Check sheet for the modelled part. Datum: model origin and axes. Units: mm. A direction names the side the tool comes from. Give positions to 0.01 mm unless a question says otherwise; leave off trailing zeros. Write each loop counter-clockwise with the first axis right and the second up, starting at its lowest first coordinate (ties: lowest second). Pieces come first, ordered by that corner, then holes. Notation, with made-up numbers: M 67,19 L 109,19 A34 ccw 109,56 Z; hole C 66,62.25 d2. An arc over 180 degrees is marked long. Write each question's results on one line, items separated by ' | '. Start each with the question number.
Autodesk Inventor part; units mm, degrees
ref_plane "YZ Plane" through (0, 0, 0) normal (1, 0, 0) x (0, 1, 0)
ref_plane "XZ Plane" through (0, 0, 0) normal (0, 1, 0) x (-1, 0, 0)
ref_plane "XY Plane" through (0, 0, 0) normal (0, 0, 1) x (1, 0, 0)
sketch "Sketch1" plane through (0, 0, 0) normal (0, 1, 0) x (-1, 0, 0)
  line L0 (0.6121, 9.4217) -> (-0.6121, 9.4217)
  line L1 (-3.6121, 6.4217) -> (-3.6121, -6.4217)
  line L2 (-0.6121, -9.4217) -> (0.6121, -9.4217)
  line L3 (3.6121, -6.4217) -> (3.6121, 6.4217)
  line L4 (3.6121, 9.4217) -> (-3.6121, -9.4217) construction
  line L5 (-3.6121, 9.4217) -> (3.6121, -9.4217) construction
  arc A0 (3.6121, 6.4217) -> (0.6121, 9.4217) centre (0.6121, 6.4217) ccw
  arc A1 (-0.6121, 9.4217) -> (-3.6121, 6.4217) centre (-0.6121, 6.4217) ccw
  arc A2 (0.6121, -9.4217) -> (3.6121, -6.4217) centre (0.6121, -6.4217) ccw
  arc A3 (-3.6121, -6.4217) -> (-0.6121, -9.4217) centre (-0.6121, -6.4217) ccw
  line L6 (2.5462, 7.5291) -> (2.5462, -7.1828) construction
  line L7 (2.5462, -7.1828) -> (-2.4754, -7.1828) construction
  line L8 (-2.4754, -7.1828) -> (-2.4754, 7.5291) construction
  line L9 (-2.4754, 7.5291) -> (2.5462, 7.5291) construction
  line L10 (0.1215, 6.8275) -> (0.1215, 5.888)
  spline S0 degree 2 poles (0.1215, 5.888) (0.1215, 5.7568) (0.2446, 5.5598) (0.4744, 5.4573) (0.6385, 5.4573) knots 0 0 0 1 2 3 3 3
  line L11 (0.6385, 5.4573) -> (1.3974, 5.4573)
  spline S1 degree 2 poles (1.3974, 5.4573) (1.5656, 5.4573) (1.8036, 5.5598) (1.9308, 5.7568) (1.9308, 5.888) knots 0 0 0 1 2 3 3 3
  line L12 (1.9308, 5.888) -> (1.9308, 6.8275)
  line L13 (1.9308, 6.8275) -> (2.5462, 6.8275)
  line L14 (2.5462, 6.8275) -> (2.5462, 5.9004)
  spline S2 degree 2 poles (2.5462, 5.9004) (2.5462, 5.5516) (2.2795, 5.0552) (1.7667, 4.7968) (1.4097, 4.7968) knots 0 0 0 1 2 3 3 3
  line L15 (1.4097, 4.7968) -> (0.6179, 4.7968)
  spline S3 degree 2 poles (0.6179, 4.7968) (0.2692, 4.7968) (-0.2313, 5.0593) (-0.4939, 5.5557) (-0.4939, 5.9004) knots 0 0 0 1 2 3 3 3
  line L16 (-0.4939, 5.9004) -> (-0.4939, 6.8275)
  line L17 (-0.4939, 6.8275) -> (0.1215, 6.8275)
  line L18 (2.5462, 7.1886) -> (2.5462, 6.5363)
  line L19 (2.5462, 6.5363) -> (-2.4221, 6.5363)
  line L20 (-2.4221, 6.5363) -> (-2.4221, 7.1886)
  line L21 (-2.4221, 7.1886) -> (2.5462, 7.1886)
  line L22 (2.5462, 3.2173) -> (2.5462, 2.6224)
  line L23 (2.5462, 2.6224) -> (-2.4221, 1.4737)
  line L24 (-2.4221, 1.4737) -> (-2.4221, 2.1711)
  line L25 (-2.4221, 2.1711) -> (1.5287, 2.9219)
  line L26 (1.5287, 2.9219) -> (-2.4221, 3.6685)
  line L27 (-2.4221, 3.6685) -> (-2.4221, 4.366)
  line L28 (-2.4221, 4.366) -> (2.5462, 3.2173)
  line L29 (-0.7277, 3.6316) -> (-0.7277, 2.1588)
  line L30 (-0.7277, 2.1588) -> (-1.339, 2.1588)
  line L31 (-1.339, 2.1588) -> (-1.339, 3.6316)
  line L32 (-1.339, 3.6316) -> (-0.7277, 3.6316)
  spline S4 degree 2 poles (-2.4713, -0.0648) (-2.4713, 0.2962) (-2.2046, 0.8049) (-1.6795, 1.0634) (-1.3062, 1.0634) knots 0 0 0 1 2 3 3 3
  line L33 (-1.3062, 1.0634) -> (2.5462, 1.0634)
  line L34 (2.5462, 1.0634) -> (2.5462, 0.4152)
  line L35 (2.5462, 0.4152) -> (-1.3308, 0.4152)
  spline S5 degree 2 poles (-1.3308, 0.4152) (-1.5769, 0.4152) (-1.8395, 0.169) (-1.8395, -0.0648) knots 0 0 0 1 2 2 2
  spline S6 degree 2 poles (-1.8395, -0.0648) (-1.8395, -0.2987) (-1.5769, -0.5489) (-1.3308, -0.5489) knots 0 0 0 1 2 2 2
  line L36 (-1.3308, -0.5489) -> (2.5462, -0.5489)
  line L37 (2.5462, -0.5489) -> (2.5462, -1.1971)
  line L38 (2.5462, -1.1971) -> (-1.3062, -1.1971)
  spline S7 degree 2 poles (-1.3062, -1.1971) (-1.6795, -1.1971) (-2.2046, -0.9346) (-2.4713, -0.4299) (-2.4713, -0.0648) knots 0 0 0 1 2 3 3 3
  line L39 (2.5462, -1.8494) -> (2.5462, -2.5018)
  line L40 (2.5462, -2.5018) -> (-2.4221, -2.5018)
  line L41 (-2.4221, -2.5018) -> (-2.4221, -1.8494)
  line L42 (-2.4221, -1.8494) -> (2.5462, -1.8494)
  line L43 (-1.8067, -2.1982) -> (-1.8067, -3.913)
  line L44 (-1.8067, -3.913) -> (-2.4221, -3.913)
  line L45 (-2.4221, -3.913) -> (-2.4221, -2.1982)
  line L46 (-2.4221, -2.1982) -> (-1.8067, -2.1982)
  line L47 (2.5462, -5.3366) -> (2.5462, -5.9315)
  line L48 (2.5462, -5.9315) -> (-2.4221, -7.0802)
  line L49 (-2.4221, -7.0802) -> (-2.4221, -6.3828)
  line L50 (-2.4221, -6.3828) -> (1.5287, -5.632)
  line L51 (1.5287, -5.632) -> (-2.4221, -4.8854)
  line L52 (-2.4221, -4.8854) -> (-2.4221, -4.1879)
  line L53 (-2.4221, -4.1879) -> (2.5462, -5.3366)
  line L54 (-0.7277, -4.9223) -> (-0.7277, -6.3951)
  line L55 (-0.7277, -6.3951) -> (-1.339, -6.3951)
  line L56 (-1.339, -6.3951) -> (-1.339, -4.9223)
  line L57 (-1.339, -4.9223) -> (-0.7277, -4.9223)
  point P0 (0, 0)
  dimension "d0" = 3
extrude "Extrusion1" add sketch "Sketch1" against normal blind 2 contours A0 L3 A2 L2 A3 L1 A1 L0 | L17 L16 L19 L20 L21 L18 L13 L12 L10 | L10 L19 L16 L17 | L19 L12 S1 L11 S0 L10 | L10 S0 L11 S1 L12 L19 L14 S2 L15 S3 L16 | L12 L13 L14 L19 | L22 L23 L24 L25 L31 L30 L29 L26 L32 L27 L28 | L31 L32 L29 L26 | L26 L29 L25 L31 | L25 L29 L30 L31 | L26 L25 L29 | S4 L33 L34 L35 S5 S6 L36 L37 L38 S7 | L39 L40 L43 L46 L41 L42 | L43 L44 L45 L40 | L40 L41 L46 L43 | L47 L48 L49 L50 L56 L55 L54 L51 L57 L52 L53 | L56 L57 L54 L51 | L51 L54 L50 L56 | L50 L54 L55 L56 | L51 L50 L54
extrude "Extrusion2" add sketch "Sketch1" along normal blind 1 contours L17 L16 L19 L20 L21 L18 L13 L12 L10 | L10 L19 L16 L17 | L10 S0 L11 S1 L12 L19 L14 S2 L15 S3 L16 | L12 L13 L14 L19 | L22 L23 L24 L25 L31 L30 L29 L26 L32 L27 L28 | L31 L32 L29 L26 | L26 L29 L25 L31 | L25 L29 L30 L31 | S4 L33 L34 L35 S5 S6 L36 L37 L38 S7 | L39 L40 L43 L46 L41 L42 | L43 L44 L45 L40 | L40 L41 L46 L43 | L47 L48 L49 L50 L56 L55 L54 L51 L57 L52 L53 | L56 L57 L54 L51 | L51 L54 L50 L56 | L50 L54 L55 L56
sketch "Sketch2" plane through (0, 0, 0) normal (0, 1, 0) x (1, 0, 0)
  circle A0 centre (0, -8.337) radius 0.4289
  circle A1 centre (0, 8.1055) radius 0.4428
  point P0 (0, 0)
extrude "Extrusion3" cut sketch "Sketch2" against normal through all
properties part number "_3DPrint"
Q1. Scan lines: L1, parallel to Z at x = 0, y = -0.85; L2, parallel to Y at x = 3, z = 0.5; L3, parallel to X at y = -0.2, z = 8.5. Record each from-to range of solid material in increasing order.
Q2. Release check for a two-part mould opening along X. For faces 1 (the face through (1.89, 0.49, -6.28)), 2 (the face through (0, -2, 0)), 3 (the face through (-0.056, -0.986, 7.912)), 4 (the face through (-0.027, 0.493, -4.754)) record: pulls with the +X half, pulls with the -X half, needs draft (parallel to the pull), parting line crosses it, or undercut.
Q3. Tool access check on faces 5 (the face through (1.87, 0.49, -4.99)), 6 (the face through (-0.6, 0.5, 0.415)), 7 (the face through (-1, 0.5, 6.536)). Record the directions out of +Z, -Z, +X, -X, +Y, -Y that give a thin tool (end or side, any length) a straight path to the whole face; none if there is none.
Q4. Section check A-A on y = 0.45. State how many separate pieces and enclosed holes the cut face has, plus the area to 3 significant figures.
Q5. Depth check by flat-ended pin: pin 1 Ø0.7 at (y, z) = (0.5, -5.5) entering from -X; pin 2 Ø1.1 at (x, y) = (1, 0.5) entering from -Z; pin 3 Ø0.8 at (y, z) = (0.5, 4) entering from +X. Enter the tip coordinate at first touch or a pass-through.
Q6. Section check B-B on z = -2.25. Record the boundary of the cut face in (x, y).
Q7. Section check D-D on x = 1. Record the boundary of the cut face in (y, z), plus the area to 3 significant figures.
Q8. Section check C-C on y = -1.3. Record the boundary of the cut face in (x, z), plus the area to 3 significant figures.
Check result:
1) L1: -9.42 to -8.55, -7.66 to 7.91, 8.77 to 9.42 | L2: -2 to 0 | L3: -2.78 to -0.4, 0.4 to 2.78
2) face 1: pulls with the +X half | face 2: needs draft | face 3: undercut | face 4: pulls with the -X half
3) face 5: +X, +Y | face 6: -X, +Y | face 7: +Y
4) separate pieces: 5 | enclosed holes: 3 | area: 29.7 mm^2
5) pin 1: x = -2.55 | pin 2: z = -9.42 | pin 3: x = 2.42
6) outline: M -3.61,-2 L 3.61,-2 L 3.61,0 L 2.42,0 L 2.42,1 L -2.55,1 L -2.55,0 L -3.61,0 Z
7) outline: M -2,-9.4 L 0,-9.4 L 0,-6.75 L 1,-6.75 L 1,-4.52 L 0,-4.52 L 0,-2.5 L 1,-2.5 L 1,-1.85 L 0,-1.85 L 0,-1.2 L 1,-1.2 L 1,-0.55 L 0,-0.55 L 0,0.42 L 1,0.42 L 1,1.06 L 0,1.06 L 0,1.8 L 1,1.8 L 1,4.04 L 0,4.04 L 0,6.54 L 1,6.54 L 1,7.19 L 0,7.19 L 0,9.4 L -2,9.4 Z | area: 44.7 mm^2
8) outline: M -3.61,-6.42 A3 ccw -0.61,-9.42 L 0.61,-9.42 A3 ccw 3.61,-6.42 L 3.61,6.42 A3 ccw 0.61,9.42 L -0.61,9.42 A3 ccw -3.61,6.42 Z; hole C 0,-8.11 d0.89; hole C 0,8.34 d0.86 | area: 127 mm^2
